from build123d import *

# Parameters (mm, degrees)
F0_R      = 55
F1_DEPTH  = 25
F2_R      = 40
F3_DEPTH  = 2
F4_R      = 11
F5_DEPTH  = 7
F6_R      = 40
F7_DEPTH  = 2
F8_R      = 11
F9_DEPTH  = 7
F10_R     = 9
F11_DEPTH = 25
F12_R     = 12.49999


# Not quite as in the source:
# - a fillet or chamfer is up to 0.001 mm smaller than in the source, because OpenCascade refuses the exact size


with BuildPart() as f1:
    # F0 (on Top) → F1 (new body)
    with BuildSketch(Plane.XY):
        Circle(F0_R)
    extrude(amount=F1_DEPTH)

    # F2 (on face) → F3 (cut)
    with BuildSketch(Plane.XY.offset(25)):
        Circle(F2_R)
    extrude(amount=-F3_DEPTH, mode=Mode.SUBTRACT)

    # F4 (on face) → F5 (cut)
    with BuildSketch(Plane.XY.offset(23)):
        Circle(F4_R)
    extrude(amount=-F5_DEPTH, mode=Mode.SUBTRACT)

    # F6 (on face) → F7 (cut)
    with BuildSketch(Plane(origin=(0, 0, 0), x_dir=(1, 0, 0), z_dir=(0, 0, -1))):
        Circle(F6_R)
    extrude(amount=-F7_DEPTH, mode=Mode.SUBTRACT)

    # F8 (on face) → F9 (cut)
    with BuildSketch(Plane(origin=(0, 0, 2), x_dir=(1, 0, 0), z_dir=(0, 0, -1))):
        Circle(F8_R)
    extrude(amount=-F9_DEPTH, mode=Mode.SUBTRACT)

    # F10 (on face) → F11 (cut)
    with BuildSketch(Plane.XY.offset(16)):
        Circle(F10_R)
    extrude(amount=-F11_DEPTH, mode=Mode.SUBTRACT)

    # F12 (radius 12.5 in the source; OpenCascade refuses exactly that, so slightly less here)
    f12_edges = [f1.edges().sort_by_distance(p)[0] for p in [
        (-55, 0, 25),
        (-55, 0, 0),
    ]]
    fillet(f12_edges, radius=F12_R)


solid = f1.part
The listing builds one solid part. Answer for the finished solid, in the listing's coordinates (mm). A direction names the side the tool comes from. Round coordinates to 2 decimals unless told otherwise and drop trailing zeros. Order: outer loops, then holes, each group sorted by start corner. A loop starts at its lowest first (then second) coordinate and runs counter-clockwise, first axis right, second up. Notation, with made-up numbers: (88.25, -29.5) -> (137.25, -29.5) arc R19 ccw to (137.25, -13.5) -> close; hole circle Ø3 at (19, 46.5). An arc over 180 degrees is marked (long way). Write each question's results on one line, items separated by ' | '. Start each with the question number.
Q1. Straight lines are drawn through the part: probe 1 along Y at (x, z) = (0, 12.5); probe 2 along X at (y, z) = (-7.5, 9.5); probe 3 along X at (y, z) = (1, 23.5). For each, find the intervals that lie inside material, in ascending order. Write a range as from..to.
Q2. Find section D-D (z = 4.5). Determine the outline of the cut face in (x, y), then the cut area to 3 significant figures.
Q3. Find section C-C (z = 18.5). Determine the outline of the cut face in (x, y), then the cut area to 3 significant figures.
Q4. Each of these flat-tipped pins is pushed along its axis until it touches: pin 1 (6 mm diameter, centred on x = -21, y = 6, fed in from +Z); pin 2 (1 mm diameter, centred on y = 6.5, z = 14, fed in from +X); pin 3 (3 mm diameter, centred on x = -29, y = 35.5, fed in from -Z); pin 4 (17.5 mm diameter, centred on x = 0, y = 0, fed in from +Z). Where does it stop, or does it pass through?
Q5. Which of the six approach directions +Z, -Z, +X, -X, +Y, -Y give full straight-line access (tool end or side, diameter ignored) to faces 1 (the flat face through (2, 9, 9)), 2 (the cylindrical face through (-2.38, -10.74, 19.55)), 3 (the cylindrical face through (-1.172, 8.923, 12.549))?
Q6. The mould has two halves that part along Y. Classify faces 4 (the flat face through (2, -9, 16)), 5 (the flat face through (-29, -28, 0)): pulls with the +Y half, pulls with the -Y half, needs draft (parallel to the pull), parting line crosses it, or undercut.
Worked answers:
1) probe 1: y = -55..-9, 9..55 | probe 2: x = -54.12..-4.97, 4.97..54.12 | probe 3: x = -48.43..-39.99, 39.99..48.43
2) outline: circle Ø104.21 at (0, 0); hole circle Ø22 at (0, 0) | area: 8,150 mm2
3) outline: circle Ø106.93 at (0, 0); hole circle Ø22 at (0, 0) | area: 8,600 mm2
4) pin 1: stops at z = 23 | pin 2: stops at x = 54.6 | pin 3: stops at z = 0.14 | pin 4: passes through
5) face 1: -Z | face 2: +Z | face 3: +Z, -Z
6) face 4: undercut | face 5: needs draft
